from build123d import *

# Parameters (mm, degrees)
F1_DEPTH = 12.7
F0_W     = 20.32
F0_H     = 25.4
F2_DEPTH = 38.1
F0_W_2   = 35.56
F3_DEPTH = 38.1
F5_DEPTH = 25.4


with BuildPart() as f1:
    # F0 (on Top) → F1 (new body)
    with BuildSketch(Plane.XY):
        Polygon((0, 50.8), (0, 0), (25.4, 0), (25.4, 12.7), (50.8, 12.7), (50.8, 0), (76.2, 0), (76.2, 25.4), (55.88, 25.4), (20.32, 25.4), (20.32, 50.8), align=None)
    extrude(amount=F1_DEPTH)

    # F0 (on Top) → F2 (join)
    with BuildSketch(Plane.XY):
        with Locations((66.04, 38.1)):
            Rectangle(F0_W, F0_H)
    extrude(amount=F2_DEPTH)

    # F0 (on Top) → F3 (join)
    with BuildSketch(Plane.XY):
        with Locations((38.1, 38.1)):
            Rectangle(F0_W_2, F0_H)
    extrude(amount=F3_DEPTH)

    # F4 (on face) → F5 (cut)
    with BuildSketch(Plane.XZ.offset(-25.4)):
        Polygon((20.32, 38.1), (20.32, 12.7), (55.88, 38.1), align=None)
    extrude(amount=-F5_DEPTH, mode=Mode.SUBTRACT)


solid = f1.part
Build history of the part. All positions in model axes, mm. A direction names the side the tool comes from. Coordinates: 2 decimals unless noted, no trailing zeros. Order: outer loops, then holes, each group sorted by start corner. A loop starts at its lowest first (then second) coordinate and runs counter-clockwise, first axis right, second up. Notation, with made-up numbers: (26, 17) - (69, 17) arc R18 ccw to (69, 51) - close; hole circle Ø6 at (59, 3). An arc over 180 degrees is marked (long way). Write item = value, one per line. Start each with the question number.
1) Two-plate mould, pull along X, no slides. Class faces 6 (the face through (63, 0, 6)), 7 (the face through (37.85, 37.92, 25.22)), 8 (the face through (50.8, 6, 6)): pulls with the +X half, pulls with the -X half, needs draft (parallel to the pull), parting line crosses it, or undercut.
2) Wall check: line 1 along X through (y, z) = (12.5, 4); line 2 along Y through (x, z) = (31, 2); line 3 along Z through (x, y) = (39.5, 20). Give the ranges that are in metal, low to high. Write a range as from..to.
3) 3-axis set-ups, long thin cutter, end or side, ignore diameter. For faces 1 (the face through (54, 25.4, 22)), 2 (the face through (29, 20, 12.7)), 3 (the face through (0, 26, 6)), 4 (the face through (25.4, 6, 6)), 5 (the face through (13, 0, 6)): which of +Z, -Z, +X, -X, +Y, -Y reach the whole face in a straight line?
4) Flat gauge pins, fed straight in: pin 1 Ø4 at (x, z) = (40.5, 7) entering from -Y; pin 2 Ø8 at (y, z) = (25, 33.5) entering from -X; pin 3 Ø8 at (y, z) = (21, 32.5) entering from -X. Where does each tip first touch, or does it go through?
5) Saw through at D-D on x = 65.5. Write the cut outline in (y, z).
6) Saw through at C-C on y = 46.5. Write the cut outline in (x, z), then the cut area to 3 significant figures.
7) Saw through at B-B on z = 6. Write the cut outline in (x, y), then the cut area to 3 significant figures.
8) Saw through at A-A on y = 7. Write the cut outline in (x, z).
From the geometry:
q1.face_6 = needs draft
q1.face_7 = pulls with the -X half
q1.face_8 = undercut
q2.line_1 = 0..25.4, 50.8..76.2
q2.line_2 = 12.7..50.8
q2.line_3 = 0..12.7
q3.face_1 = +Z, +X, -X, -Y
q3.face_2 = +Z, -X, -Y
q3.face_3 = +Z, -Z, -X, +Y, -Y
q3.face_4 = +Z, -Z, -Y
q3.face_5 = +Z, -Z, +X, -X, -Y
q4.pin_1 = 12.7
q4.pin_2 = 43.87
q4.pin_3 = through
q5.outline = (0, 0) - (50.8, 0) - (50.8, 38.1) - (25.4, 38.1) - (25.4, 12.7) - (0, 12.7) - close
q6.outline = (0, 0) - (76.2, 0) - (76.2, 38.1) - (55.88, 38.1) - (20.32, 12.7) - (0, 12.7) - close
q6.area = 1,940 mm^2
q7.outline = (0, 0) - (25.4, 0) - (25.4, 12.7) - (50.8, 12.7) - (50.8, 0) - (76.2, 0) - (76.2, 50.8) - (0, 50.8) - close
q7.area = 3,550 mm^2
q8.outline = (0, 0) - (25.4, 0) - (25.4, 12.7) - (0, 12.7) - close; (50.8, 0) - (76.2, 0) - (76.2, 12.7) - (50.8, 12.7) - close
